```python
from build123d import *

# Parameters (mm, degrees)
F0_W            = 88.9
F0_H            = 88.9
F1_DEPTH        = 6.35
F2_R            = 9.525
F3_DEPTH        = 38.1
F4_W            = 38.1
F4_H            = 20.32
F5_DEPTH        = 5.08
F6_R            = 3.175
F7_DEPTH        = 10.16
F7_DEPTH_BACK   = 2.54
F7_COPIES_COUNT = 4
F8_W            = 6.35
F8_H            = 6.35
F9_DEPTH        = 6.35


# Not quite as in the source:
# - a pattern or mirror of a feature is missing from the dataset's text; its kind, count and spacing are read off the source's solid


with BuildPart() as f1:
    # F0 (on Top) → F1 (new body)
    with BuildSketch(Plane.XY):
        Rectangle(F0_W, F0_H)
    extrude(amount=F1_DEPTH)

    # F2 (on face) → F3 (join)
    with BuildSketch(Plane.XY.offset(6.35)):
        Circle(F2_R)
    extrude(amount=F3_DEPTH)

    # F4 (on face) → F5 (join)
    with BuildSketch(Plane.XY.offset(6.35)):
        with Locations((0, 26.67)):
            Rectangle(F4_W, F4_H)
    extrude(amount=F5_DEPTH)

    # F6 (on face) → F7 (join, two sides)
    with BuildSketch(Plane.XY.offset(6.35)) as f7_sk:
        with Locations((-34.925, 34.925)):
            Circle(F6_R)
    f7 = extrude(amount=-F7_DEPTH) + extrude(f7_sk.sketch, amount=F7_DEPTH_BACK)

    # F7_copies: F7 ×4 about axis
    f7_copies_axis = Axis((0, 0, 0), (0, 0, 1))
    for i in range(1, F7_COPIES_COUNT):
        add(f7.rotate(f7_copies_axis, i * 360 / F7_COPIES_COUNT))

    # F8 (on face) → F9 (cut)
    with BuildSketch(Plane.XY.offset(6.35)):
        with Locations((0, -41.275)):
            Rectangle(F8_W, F8_H)
    extrude(amount=-F9_DEPTH, mode=Mode.SUBTRACT)


solid = f1.part
```
Geometry check sheet. Reference: the model listing, model coordinates, mm. A direction names the side the tool comes from. Coordinates: 2 decimals unless noted, no trailing zeros. Write each loop counter-clockwise with the first axis right and the second up, starting at its lowest first coordinate (ties: lowest second). Pieces come first, ordered by that corner, then holes. Notation, with made-up numbers: M 83.25,59.25 L 134.25,59.25 A18 cw 134.25,92.25 Z; hole C -22.75,19 d6. An arc over 180 degrees is marked long. Use one line per item in the form item = value. Start each with the question number.
1) Go/stop test with flat-tipped pins: pin 1 Ø5 at (x, y) = (33.5, -34) entering from +Z; pin 2 Ø1.9 at (x, z) = (1, 3) entering from -Y; pin 3 Ø2.5 at (y, z) = (23.5, 10) entering from +X. Record where each tip stops, or that it passes through.
2) Release check for a two-part mould opening along Y. For faces 1 (the cylindrical face through (-37.602, -33.218, -1.878)), 2 (the flat face through (-1, 44.45, 3)), 3 (the flat face through (0, 27, 11.43)) record: pulls with the +Y half, pulls with the -Y half, needs draft (parallel to the pull), parting line crosses it, or undercut.
3) Set-up check for faces 4 (the cylindrical face through (33.218, -37.602, 7.638)), 5 (the cylindrical face through (-33.218, 37.602, -1.878)), 6 (the flat face through (0, 36.83, 9)), 7 (the flat face through (3.175, -41, 3)): record each of +Z, -Z, +X, -X, +Y, -Y from which the full face is reachable in a straight line by a thin tool's end or side.
4) Section check C-C on z = 38. Enter the section's corners in (x, y) (3 decimals), and give its area (3 significant figures).
5) Thickness scan on probe 1 along X at (y, z) = (-40, 4) (3 decimals); probe 2 along Z at (x, y) = (-37, 38); probe 3 along Y at (x, z) = (6, 10). Record the ranges inside material, lowest first. Write a range as from..to.
6) Section check B-B on y = 30.5. Enter the section's corners in (x, z), and give its area (3 significant figures).
7) Section check A-A on x = 16. Enter the section's corners in (y, z).
8) Section check D-D on x = 0. Enter the section's corners in (y, z) (3 decimals), and give its area (3 significant figures).
Responses:
q1.pin_1 = 8.89
q1.pin_2 = -38.1
q1.pin_3 = 19.05
q2.face_1 = undercut
q2.face_2 = pulls with the +Y half
q2.face_3 = needs draft
q3.face_4 = +Z
q3.face_5 = -Z
q3.face_6 = +Z, +Y
q3.face_7 = +Z, -Z, -Y
q4.outline = C 0,0 d19.05
q4.area = 285 mm2
q5.probe_1 = -44.45..-3.175, 3.175..44.45
q5.probe_2 = 0..6.35
q5.probe_3 = -7.4..7.4, 16.51..36.83
q6.outline = M -44.45,0 L 44.45,0 L 44.45,6.35 L 19.05,6.35 L 19.05,11.43 L -19.05,11.43 L -19.05,6.35 L -44.45,6.35 Z
q6.area = 758 mm2
q7.outline = M -44.45,0 L 44.45,0 L 44.45,6.35 L 36.83,6.35 L 36.83,11.43 L 16.51,11.43 L 16.51,6.35 L -44.45,6.35 Z
q8.outline = M -38.1,0 L 44.45,0 L 44.45,6.35 L 36.83,6.35 L 36.83,11.43 L 16.51,11.43 L 16.51,6.35 L 9.525,6.35 L 9.525,44.45 L -9.525,44.45 L -9.525,6.35 L -38.1,6.35 Z
q8.area = 1,350 mm2
